Check sheet for the drawn part. Datum: minimum x, y, z corner. Units: mm. Round coordinates to 2 decimals unless told otherwise and drop trailing zeros. Write each loop counter-clockwise with the first axis right and the second up, starting at its lowest first coordinate (ties: lowest second). Pieces come first, ordered by that corner, then holes. Notation, with made-up numbers: M 51.25,-4.75 L 73.25,-4.75 A18 cw 73.25,3.25 Z; hole C -22.75,44.25 d11. An arc over 180 degrees is marked long. One line per item, written item: value.
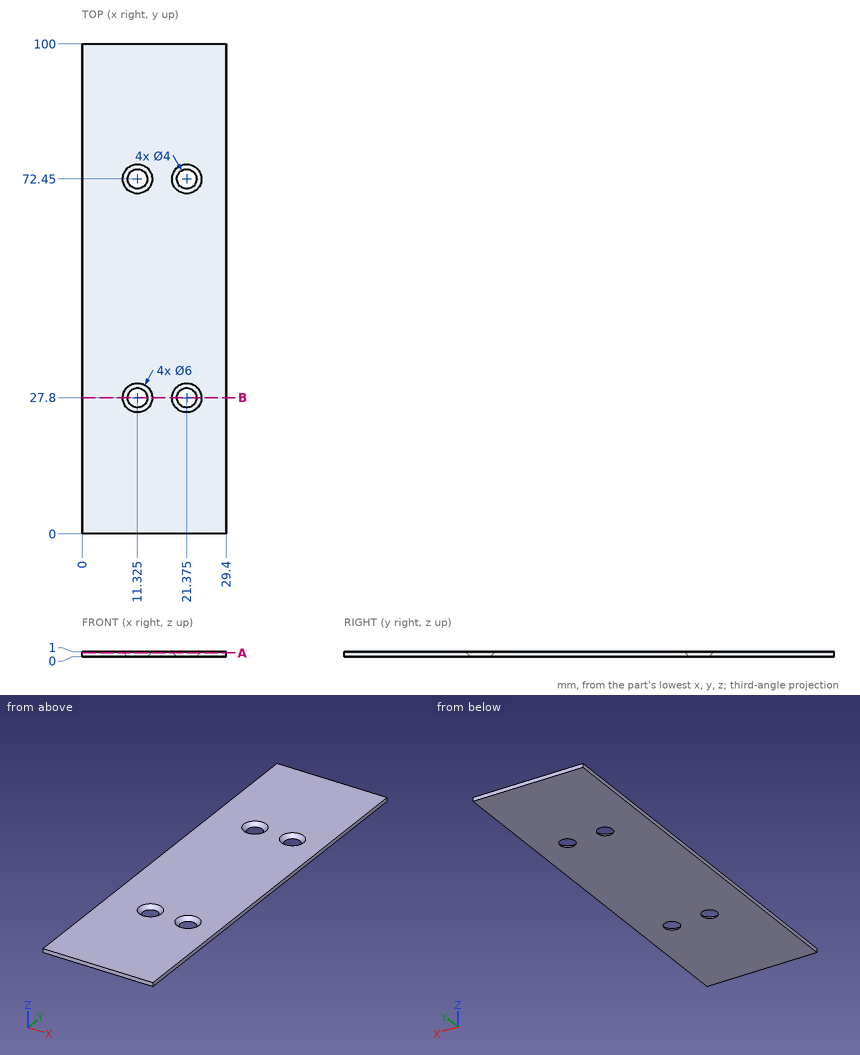
Q1. Sectioned sample at B-B on y = 27.8. Enter the section's corners in (x, z) (3 decimals).
Completed:
outline: M 0,0 L 9.325,0 L 8.325,1 L 0,1 Z; M 13.325,0 L 19.375,0 L 18.375,1 L 14.325,1 Z; M 23.375,0 L 29.4,0 L 29.4,1 L 24.375,1 Z
Q2. Sectioned sample at A-A on z = 0.8. Enter the section's corners in (x, y) (3 decimals), and give its area (3 significant figures).
Completed:
outline: M 0,0 L 29.4,0 L 29.4,100 L 0,100 Z; hole C 11.325,27.8 d5.6; hole C 11.325,72.45 d5.6; hole C 21.375,27.8 d5.6; hole C 21.375,72.45 d5.6
area: 2,840 mm^2
Q3. Scan lines: line 1 (Y direction, x = 12.75, z = 0.65); line 2 (Y direction, x = 23.5, z = 0.4); line 3 (X direction, y = 29.5, z = 0.6). Record each from-to range of solid material in increasing order. Write a range as [from, to].
Completed:
line 1: [0, 25.57], [30.03, 70.22], [74.68, 100]
line 2: [0, 26.68], [28.92, 71.33], [73.57, 100]
line 3: [0, 9.36], [13.29, 19.41], [23.34, 29.4]
